Here's how the part is built. I have some questions about the finished solid (model axes, mm). A direction names the side the tool comes from. Round coordinates to 2 decimals unless told otherwise and drop trailing zeros. Loops run counter-clockwise (first coordinate to the right, second up) from the corner with the lowest first, then second, coordinate; pieces in that order, holes last. Notation, with made-up numbers: M 87,48.5 L 103,48.5 A6 cw 103,53.5 Z; hole C 72,14.25 d1. An arc over 180 degrees is marked long. Answer as a JSON object with one key per item and string values.
from build123d import *

# Parameters (mm, degrees)
SKETCH1_R                     = 17.78
BOSS_EXTRUDE1_DEPTH           = 50.8
SHELL1_T                      = -2.54
SKETCH2_R                     = 3.175
CUT_EXTRUDE1_DEPTH            = 55.417684625
TAP_DRILL_FOR_0_80_TAP1_D     = 3.175
TAP_DRILL_FOR_0_80_TAP1_DEPTH = 6.35
TAP_DRILL_FOR_0_80_TAP1_TIP   = 1.332070664
CIRPATTERN1_COUNT             = 3


with BuildPart() as part:
    # Sketch1 → Boss-Extrude1 (new body)
    with BuildSketch(Plane(origin=(0, 0, 0), x_dir=(1, 0, 0), z_dir=(0, 1, 0))):
        with Locations(Location((0, 0, 0), (0, 0, 270))):
            Circle(SKETCH1_R)
    extrude(amount=BOSS_EXTRUDE1_DEPTH)

    # Shell1
    shell1_openings = [part.faces().sort_by_distance(p)[0] for p in [
        (0, 0, 0),
    ]]
    offset(amount=SHELL1_T, openings=shell1_openings, kind=Kind.INTERSECTION)

    # Sketch2 → Cut-Extrude1 (cut, through all)
    with BuildSketch(Plane.XZ.offset(-48.26)):
        with Locations(Location((0, 0, 0), (0, 0, 270))):
            Circle(SKETCH2_R)
    extrude(amount=-CUT_EXTRUDE1_DEPTH, mode=Mode.SUBTRACT)

    # Tap Drill for #0-80 Tap1
    with Locations(Plane(origin=(-0.363072826, 46.659447592, 17.776292587), x_dir=(0.999791484059, 0, 0.0204202939), z_dir=(-0.0204202939, 0, 0.999791484059))):
        with Locations((0, 0)):
            Hole(TAP_DRILL_FOR_0_80_TAP1_D / 2, depth=TAP_DRILL_FOR_0_80_TAP1_DEPTH)
            with Locations((0, 0, -(TAP_DRILL_FOR_0_80_TAP1_DEPTH + TAP_DRILL_FOR_0_80_TAP1_TIP / 2))):  # 100° drill point
                Cone(0, TAP_DRILL_FOR_0_80_TAP1_D / 2, TAP_DRILL_FOR_0_80_TAP1_TIP, mode=Mode.SUBTRACT)

    # Sketch8 → Tap Drill for #2-56 Tap1 (revolve, cut)
    with BuildSketch(Plane(origin=(-2.247699143, 7.424974445, 17.637353786), x_dir=(0.9919771533037619, 0, 0.1264172746240199), z_dir=(0, 1, 0))):
        Polygon((0, 0), (0, 9.635959572), (0.889, 8.89), (0.889, 0), align=None)
    tap_drill_for_2_56_tap1 = revolve(axis=Axis((-3.050448837, 7.424974445, 23.936408709), (0.1264172746240199, 0, -0.9919771533037619)), mode=Mode.SUBTRACT)

    # CirPattern1: Tap Drill for #2-56 Tap1 ×3 about axis
    cirpattern1_axis = Axis((0, 50.8, 0), (0, -1, 0))
    for i in range(1, CIRPATTERN1_COUNT):
        add(tap_drill_for_2_56_tap1.rotate(cirpattern1_axis, i * 360 / CIRPATTERN1_COUNT), mode=Mode.SUBTRACT)


solid = part.part
Item 1: If I drill on L1, parallel to X at y = 18, z = 0; L2, parallel to Z at x = 13.5, y = 22; L3, parallel to X at y = 34.5, z = -14, over which ranges is the centre line in solid material (lowest first)? Write a range as from..to.
Solution:
{"L1": "x = -17.78..-15.24, 15.24..17.78", "L2": "z = -11.57..-7.07, 7.07..11.57", "L3": "x = -10.96..-6.02, 6.02..10.96"}
Item 2: We'd pull the mould along Y, two halves only. Please class faces 3 (the face through (-4, 50.8, 0)), 4 (the face through (-1.93, 49.51, 2.52)), 5 (the face through (15.306, 8.293, -6.205)), 6 (the face through (-2.279, 8.293, 16.358)): +Y half, -Y half, draft (parallel to the pull), parting line (faces both ways), or undercut.
Solution:
{"face 3": "+Y half", "face 4": "draft", "face 5": "undercut", "face 6": "undercut"}
Item 3: For faces 1 (the face through (-13.027, 8.293, -10.153)), 2 (the face through (15.11, 23.8, -1.98)), which set-ups out of +Z, -Z, +X, -X, +Y, -Y let a thin tool reach every point of the face, with its end or its side?
Solution:
{"face 1": "none", "face 2": "-Y"}
Item 4: I want a section at C-C on y = 4.5. List the corners of the cut face in (x, z) for me, plus the area to 3 significant figures.
Solution:
{"outline": "C 0,0 d35.56; hole C 0,0 d30.48", "area": "263 mm2"}
Item 5: For P1, Ø9, axis at x = 2.5, z = 0, coming from the -Y side; P2, Ø1, axis at x = -13, y = 7, coming from the +Z side; P3, Ø6, axis at x = 3.5, y = 6.5, coming from the +Z side; P4, Ø2, axis at y = 37.5, z = 1, coming from the -X side, each with a flat end and sliding along its axis, tell me the tip position at first contact or that it passes through.
Solution:
{"P1": "stops at y = 48.26", "P2": "stops at z = 12.64", "P3": "stops at z = 17.77", "P4": "stops at x = -17.78"}
Item 6: I want a section at D-D on x = -7. List the corners of the cut face in (y, z) for me, plus the area to 3 significant figures.
Solution:
{"outline": "M 0,-16.34 L 50.8,-16.34 L 50.8,16.34 L 0,16.34 L 0,13.54 L 48.26,13.54 L 48.26,-13.54 L 0,-13.54 Z", "area": "354 mm2"}
Item 7: I want a section at A-A on z = 0. List the corners of the cut face in (x, y) for me (3 decimals).
Solution:
{"outline": "M -17.78,0 L -15.24,0 L -15.24,48.26 L -3.175,48.26 L -3.175,50.8 L -17.78,50.8 Z; M 3.175,48.26 L 15.24,48.26 L 15.24,0 L 17.78,0 L 17.78,50.8 L 3.175,50.8 Z"}
Item 8: I want a section at B-B on z = 7.5. List the corners of the cut face in (x, y) for me, plus the area to 3 significant figures.
Solution:
{"outline": "M -16.12,0 L -13.27,0 L -13.27,48.26 L 13.27,48.26 L 13.27,0 L 16.12,0 L 16.12,50.8 L -16.12,50.8 Z", "area": "357 mm2"}
